Input: part model. Units: mm. Frame: model coordinates. Coordinates: 2 decimals unless noted, no trailing zeros. Write each loop counter-clockwise with the first axis right and the second up, starting at its lowest first coordinate (ties: lowest second). Pieces come first, ordered by that corner, then holes. Notation, with made-up numbers: (30, -3) - (72, -3) arc R33 ccw to (72, 34) - close; hole circle Ø7 at (-9, -4). An arc over 180 degrees is marked (long way). Put each result on its own line as item: value. Start each with the question number.
1. Cut plane D-D, the plane z = -0.75. Return loops of the section in (x, y).
2. Cut plane A-A, the plane z = -6.35. Return loops of the section in (x, y), and give its area (3 significant figures).
3. Cut plane C-C, the plane y = 83.5. Return loops of the section in (x, z).
4. Cut plane B-B, the plane x = -105. Return loops of the section in (y, z).
5. Line query: line 1 (Y direction, x = -104.25, z = -6.35); line 2 (Y direction, x = -101.5, z = -6.35); line 3 (Z direction, x = -94.5, y = 82.25). Output: solid intervals per line, ascending.
6. Pull-direction query (Y, two-part tool) for faces 1 (the flat face through (-99, 82, -12.7)), 2 (the cylindrical face through (-96.136, 83.873, -6.187)), 3 (the flat face through (-99.314, 82, -6)), 4 (the flat face through (-95.68, 79.2, -11.91)); classes: released by +Y, released by -Y, zero draft, split by the parting line, or undercut.
7. Pin query (flat end, axial travel): pin 1 (7 mm diameter, centred on y = 79.38, z = -6.35, fed in from +X); pin 2 (1.5 mm diameter, centred on y = 70.5, z = -1.5, fed in from +X); pin 3 (3 mm diameter, centred on x = -102, z = -3.5, fed in from -Y). Return the tip coordinate at first contact, or that it passes through.
from build123d import *

# Parameters (mm, degrees)
BOSS_EXTRUDE2_DEPTH = 12.7
SKETCH5_R           = 2.25
CUT_EXTRUDE1_DEPTH  = 26.4
SKETCH6_R           = 4.5
CUT_EXTRUDE2_DEPTH  = 17.51


with BuildPart() as part:
    # xs → Boss-Extrude2 (new body)
    with BuildSketch(Plane.XY):
        Polygon((-108.204482014, 92.076361751), (-108.204482014, 66.676361751), (-82.804482014, 92.076361751), align=None)
    extrude(amount=-BOSS_EXTRUDE2_DEPTH)

    # Sketch5 → Cut-Extrude1 (cut, through all)
    with BuildSketch(Plane.ZY.offset(108.204482014)):
        with Locations((-6.35, 79.376361751)):
            Circle(SKETCH5_R)
    extrude(amount=-CUT_EXTRUDE1_DEPTH, mode=Mode.SUBTRACT)

    # Sketch6 → Cut-Extrude2 (cut, through all)
    with BuildSketch(Plane.ZY.offset(99.314482014)):
        with Locations((-6.35, 79.376361751)):
            Circle(SKETCH6_R)
    extrude(amount=-CUT_EXTRUDE2_DEPTH, mode=Mode.SUBTRACT)


solid = part.part
Report:
1. outline: (-108.2, 66.68) - (-82.8, 92.08) - (-108.2, 92.08) - close
2. outline: (-108.2, 66.68) - (-99.31, 75.57) - (-99.31, 77.13) - (-108.2, 77.13) - close; (-108.2, 81.63) - (-99.31, 81.63) - (-99.31, 83.88) - (-91, 83.88) - (-82.8, 92.08) - (-108.2, 92.08) - close
2. area: 248 mm^2
3. outline: (-108.2, -12.7) - (-91.38, -12.7) - (-91.38, -8.15) - (-99.31, -8.15) - (-99.31, -4.55) - (-91.38, -4.55) - (-91.38, 0) - (-108.2, 0) - close
4. outline: (69.88, -12.7) - (92.08, -12.7) - (92.08, 0) - (69.88, 0) - close; hole circle Ø4.5 at (79.38, -6.35)
5. line 1: y = 70.63 to 77.13, 81.63 to 92.08
5. line 2: y = 73.38 to 77.13, 81.63 to 92.08
5. line 3: z = -12.7 to -9.81, -2.89 to 0
6. face 1: zero draft
6. face 2: undercut
6. face 3: undercut
6. face 4: released by -Y
7. pin 1: stops at x = -99.31
7. pin 2: stops at x = -103.63
7. pin 3: stops at y = 71.38
